Verification items for the finished model (mm, model axes). Give positions to 0.01 mm unless a question says otherwise; leave off trailing zeros. Write each loop counter-clockwise with the first axis right and the second up, starting at its lowest first coordinate (ties: lowest second). Pieces come first, ordered by that corner, then holes. Notation, with made-up numbers: (25.25, -21) - (41.25, -21) arc R9 ccw to (41.25, -16) - close; hole circle Ø6 at (80.25, 50). An arc over 180 degrees is marked (long way). Put each result on its own line as item: value.
from build123d import *

# Parameters (mm, degrees)
SKETCH1_W           = 28
SKETCH1_H           = 75
BOSS_EXTRUDE1_DEPTH = 3
SKETCH2_R           = 1.05
CUT_EXTRUDE1_DEPTH  = 41.140378673
FILLET1_R           = 5


with BuildPart() as part:
    # Sketch1 → Boss-Extrude1 (new body)
    with BuildSketch(Plane.XY):
        Rectangle(SKETCH1_W, SKETCH1_H)
    extrude(amount=BOSS_EXTRUDE1_DEPTH)

    # Sketch2 → Cut-Extrude1 (cut, through all)
    with BuildSketch(Plane.XY.offset(3)):
        with Locations((-3.4, 33.5)):
            Circle(SKETCH2_R)
        with Locations((3.4, 33.5)):
            Circle(SKETCH2_R)
        with BuildLine():
            Line((-10.499999957, 12.5), (-10.499999957, 24.5))
            ThreePointArc((-10.499999957, 24.5), (-6.5, 28.499999957), (-2.500000043, 24.5))
            Line((-2.500000043, 24.5), (-2.500000043, 12.5))
            ThreePointArc((-2.500000043, 12.5), (-6.5, 8.500000043), (-10.499999957, 12.5))
        make_face()
        with BuildLine():
            Line((2.500000043, 12.5), (2.500000043, 24.5))
            ThreePointArc((2.500000043, 24.5), (6.5, 28.499999957), (10.499999957, 24.5))
            Line((10.499999957, 24.5), (10.499999957, 12.5))
            ThreePointArc((10.499999957, 12.5), (6.5, 8.500000043), (2.500000043, 12.5))
        make_face()
        with BuildLine():
            Line((-9.4, -32.5), (-9.4, -12.5))
            ThreePointArc((-9.4, -12.5), (-7.2, -10.3), (-5, -12.5))
            Line((-5, -12.5), (-5, -32.5))
            ThreePointArc((-5, -32.5), (-7.2, -34.7), (-9.4, -32.5))
        make_face()
        with BuildLine():
            Line((5, -32.5), (5, -12.5))
            ThreePointArc((5, -12.5), (7.2, -10.3), (9.4, -12.5))
            Line((9.4, -12.5), (9.4, -32.5))
            ThreePointArc((9.4, -32.5), (7.2, -34.7), (5, -32.5))
        make_face()
    extrude(amount=-CUT_EXTRUDE1_DEPTH, mode=Mode.SUBTRACT)

    # Fillet1
    fillet1_edges = [part.edges().sort_by_distance(p)[0] for p in [
        (-14, 37.5, 1.5),
        (14, 37.5, 1.5),
        (14, -37.5, 1.5),
        (-14, -37.5, 1.5),
    ]]
    fillet(fillet1_edges, radius=FILLET1_R)


solid = part.part
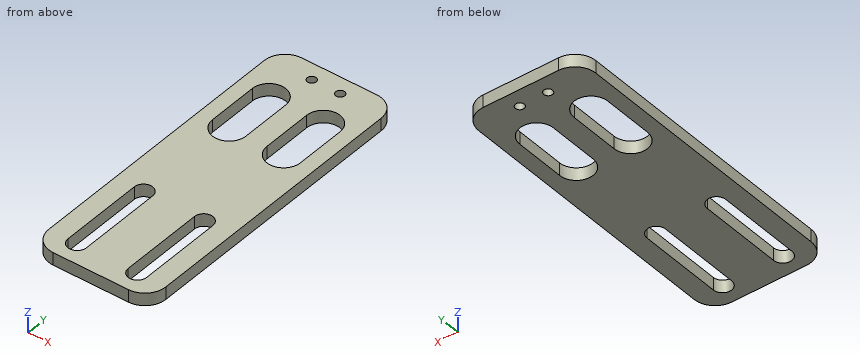
Q1. Section check A-A, the plane y = -25.5. Record the cut outline in (x, z), plus the area to 3 significant figures.
Answers follow:
outline: (-14, 0) - (-9.4, 0) - (-9.4, 3) - (-14, 3) - close; (-5, 0) - (5, 0) - (5, 3) - (-5, 3) - close; (9.4, 0) - (14, 0) - (14, 3) - (9.4, 3) - close
area: 57.6 mm2
Q2. Scan lines: line 1 along X through (y, z) = (22.5, 2.35); line 2 along X through (y, z) = (-13.5, 2.45); line 3 along Y through (x, z) = (-3.4, 0.85). Record each from-to range of solid material in increasing order.
Answers follow:
line 1: x = -14 to -10.5, -2.5 to 2.5, 10.5 to 14
line 2: x = -14 to -9.4, -5 to 5, 9.4 to 14
line 3: y = -37.5 to 9.97, 27.03 to 32.45, 34.55 to 37.5
Q3. Section check B-B, the plane z = 1.7. Record the cut outline in (x, y).
Answers follow:
outline: (-14, -32.5) arc R5 ccw to (-9, -37.5) - (9, -37.5) arc R5 ccw to (14, -32.5) - (14, 32.5) arc R5 ccw to (9, 37.5) - (-9, 37.5) arc R5 ccw to (-14, 32.5) - close; hole (-10.5, 12.5) arc R4 ccw to (-2.5, 12.5) - (-2.5, 24.5) arc R4 ccw to (-10.5, 24.5) - close; hole (-9.4, -32.5) arc R2.2 ccw to (-5, -32.5) - (-5, -12.5) arc R2.2 ccw to (-9.4, -12.5) - close; hole circle Ø2.1 at (-3.4, 33.5); hole circle Ø2.1 at (3.4, 33.5); hole (2.5, 12.5) arc R4 ccw to (10.5, 12.5) - (10.5, 24.5) arc R4 ccw to (2.5, 24.5) - close; hole (5, -32.5) arc R2.2 ccw to (9.4, -32.5) - (9.4, -12.5) arc R2.2 ccw to (5, -12.5) - close
Q4. Section check C-C, the plane x = 7.2. Record the cut outline in (y, z), plus the area to 3 significant figures.
Answers follow:
outline: (-37.5, 0) - (-34.7, 0) - (-34.7, 3) - (-37.5, 3) - close; (-10.3, 0) - (8.56, 0) - (8.56, 3) - (-10.3, 3) - close; (28.44, 0) - (37.5, 0) - (37.5, 3) - (28.44, 3) - close
area: 92.2 mm2
